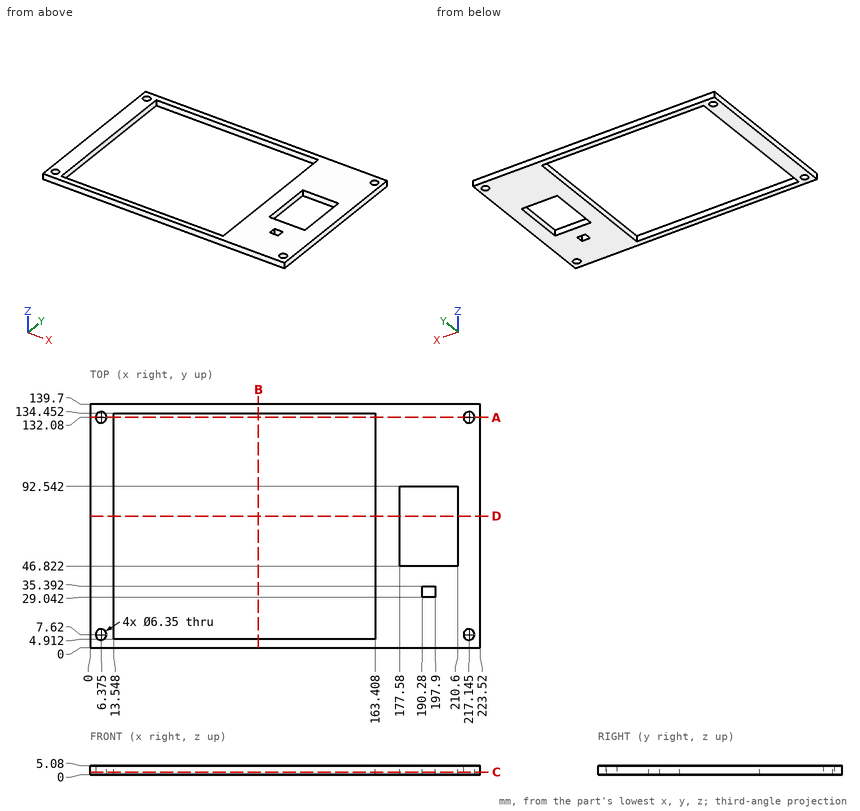
Here's the drawing with two shaded views (mm, measured from the low corner). I have some questions. Coordinates: 2 decimals unless noted, no trailing zeros. Write each loop counter-clockwise with the first axis right and the second up, starting at its lowest first coordinate (ties: lowest second). Pieces come first, ordered by that corner, then holes. Notation, with made-up numbers: M 69,-20.75 L 75,-20.75 A10 ccw 75,-9.75 Z; hole C 2.25,41.25 d2. An arc over 180 degrees is marked long. Answer as CSV lines item,"result".
Item 1: Imagine slicing it at C-C on z = 1.55. State how many separate pieces and enclosed holes the cut face has, plus the area to 3 significant figures.
Geometry results:
separate pieces,"1"
enclosed holes,"7"
area,"10,100 mm2"
Item 2: Imagine slicing it at A-A on y = 132.08. List the corners of the cut face in (x, z) for me.
Geometry results:
outline,"M 0,0 L 3.2,0 L 3.2,5.08 L 0,5.08 Z; M 9.55,0 L 13.55,0 L 13.55,5.08 L 9.55,5.08 Z; M 163.41,0 L 213.97,0 L 213.97,5.08 L 163.41,5.08 Z; M 220.32,0 L 223.52,0 L 223.52,5.08 L 220.32,5.08 Z"
Item 3: Please list where these lines run through material, in increasing order: line 1 along X through (y, z) = (132.08, 2.5); line 2 along X through (y, z) = (56, 0.55); line 3 along Y through (x, z) = (45.5, 4).
Geometry results:
line 1,"x = 0 to 3.2, 9.55 to 13.55, 163.41 to 213.97, 220.32 to 223.52"
line 2,"x = 0 to 13.55, 163.41 to 177.58, 210.6 to 223.52"
line 3,"y = 0 to 4.91, 134.45 to 139.7"
Item 4: Imagine slicing it at B-B on x = 96.5. List the corners of the cut face in (y, z) for me.
Geometry results:
outline,"M 0,0 L 4.91,0 L 4.91,5.08 L 0,5.08 Z; M 134.45,0 L 139.7,0 L 139.7,5.08 L 134.45,5.08 Z"
Item 5: I'm going to push a flat-ended pin straight in: P1, Ø4, axis at x = 217.14, y = 7.62, coming from the +Z side. Where does the tip first touch, or does it pass through?
Geometry results:
P1,"passes through"
Item 6: Imagine slicing it at D-D on y = 75.5. List the corners of the cut face in (x, z) for me.
Geometry results:
outline,"M 0,0 L 13.55,0 L 13.55,5.08 L 0,5.08 Z; M 163.41,0 L 177.58,0 L 177.58,5.08 L 163.41,5.08 Z; M 210.6,0 L 223.52,0 L 223.52,5.08 L 210.6,5.08 Z"
